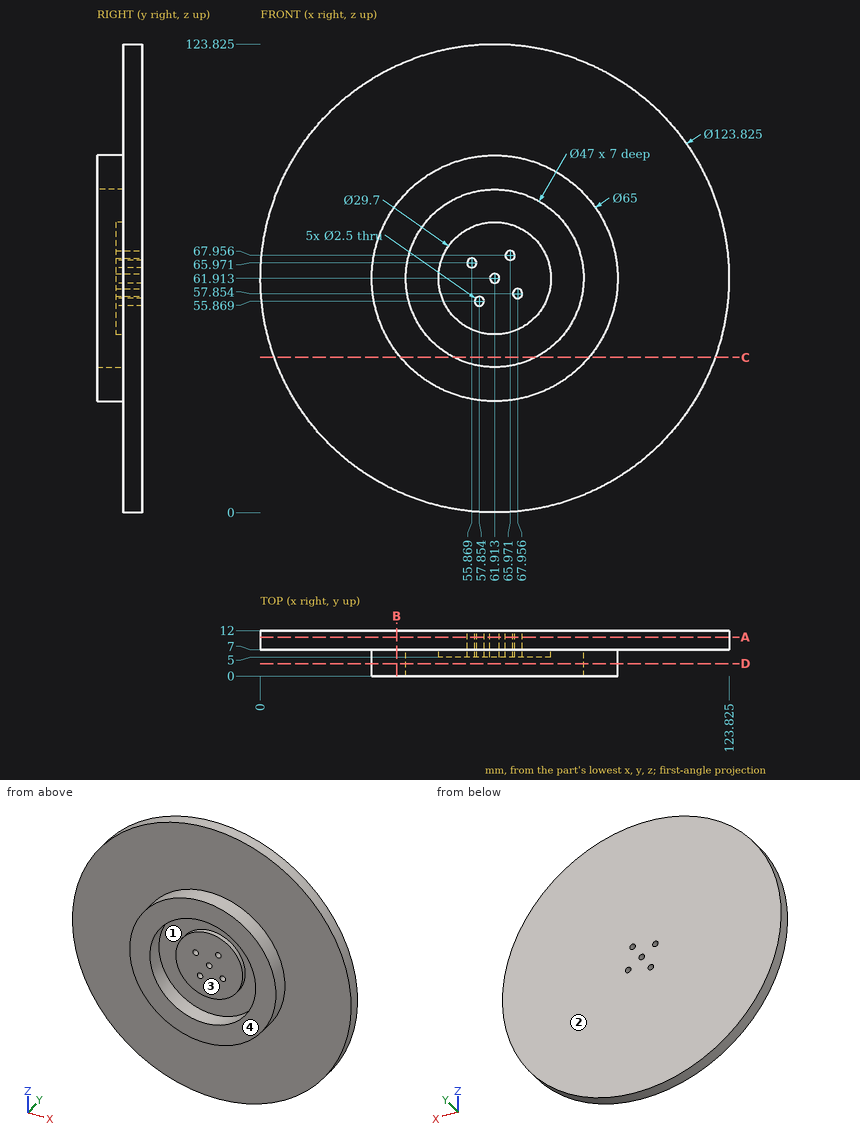
Job drawing, mm, ordinate dimensions from the low corner. One solid piece. A direction names the side the tool comes from. Give positions to 0.01 mm unless a question says otherwise; leave off trailing zeros. Loops run counter-clockwise (first coordinate to the right, second up) from the corner with the lowest first, then second, coordinate; pieces in that order, holes last. Notation, with made-up numbers: (89, 88.25) -> (104, 88.25) arc R7 cw to (104, 95.25) -> close; hole circle Ø10 at (42.25, -21). An arc over 180 degrees is marked (long way). Write each question's results on one line, items separated by ' | '. Start each with the question number.
Q1. Which spindle directions (+Z, -Z, +X, -X, +Y, -Y) get a long thin tool onto all of the face, cutting with end or side? Do the marked faces 3 and 4. Say none if no direction does.
Q2. Band-saw the part on B-B on x = 36. List the corners of the cut face in (y, z).
Q3. Pull direction X, two halves, no side cores. Call the marked faces 1 and 2: +X half, -X half, draft (parallel to the pull), parting line (faces both ways), or undercut.
Q4. Band-saw the part on A-A on y = 10.25. Count the separate pieces of the cut face and the enclosed holes in it, plus the area to 3 significant figures.
Q5. Wall check: L1, parallel to Y at x = 13.5, z = 99; L2, parallel to Y at x = 69, z = 49; L3, parallel to Z at x = 53, y = 3 (1 decimal). Give the ranges that are in metal, low to high.
Q6. Pin check, flat tips, straight feed: P1, Ø1, axis at x = 82.5, y = 10, coming from the -Z side; P2, Ø4, axis at x = 65.97, z = 67.96, coming from the -Y side; P3, Ø1, axis at y = 5.5, z = 81, coming from the +X side. Stop position of each tip, or through.
Q7. Band-saw the part on D-D on y = 3.25. List the corners of the cut face in (x, z).
Q8. Band-saw the part on C-C on z = 41. List the corners of the cut face in (x, y) (1 decimal), plus the area to 3 significant figures.
Results are:
1) face 3: -Y | face 4: +Z, -Z, +X, -X, -Y
2) outline: (0, 42.3) -> (7, 42.3) -> (7, 5.68) -> (12, 5.68) -> (12, 118.14) -> (7, 118.14) -> (7, 81.53) -> (0, 81.53) -> close
3) face 1: undercut | face 2: draft
4) separate pieces: 1 | enclosed holes: 5 | area: 12,000 mm²
5) L1: y = 7 to 12 | L2: y = 5 to 12 | L3: z = 30.7 to 40.2, 83.7 to 93.2
6) P1: stops at z = 3.35 | P2: stops at y = 5 | P3: stops at x = 88.57
7) outline: circle Ø65 at (61.91, 61.91); hole circle Ø47 at (61.91, 61.91)
8) outline: (3.6, 7) -> (37, 7) -> (37, 0) -> (51.2, 0) -> (51.2, 7) -> (72.6, 7) -> (72.6, 0) -> (86.8, 0) -> (86.8, 7) -> (120.2, 7) -> (120.2, 12) -> (3.6, 12) -> close | area: 781 mm²
